Check sheet for the drawn part. Datum: minimum x, y, z corner. Units: mm. A direction names the side the tool comes from. Round coordinates to 2 decimals unless told otherwise and drop trailing zeros. Write each loop counter-clockwise with the first axis right and the second up, starting at its lowest first coordinate (ties: lowest second). Pieces come first, ordered by that corner, then holes. Notation, with made-up numbers: (0, 52.5) -> (18, 52.5) arc R35 ccw to (18, 86.5) -> close; hole circle Ø11 at (47, 50). An arc over 180 degrees is marked (long way). One line per item, written item: value.
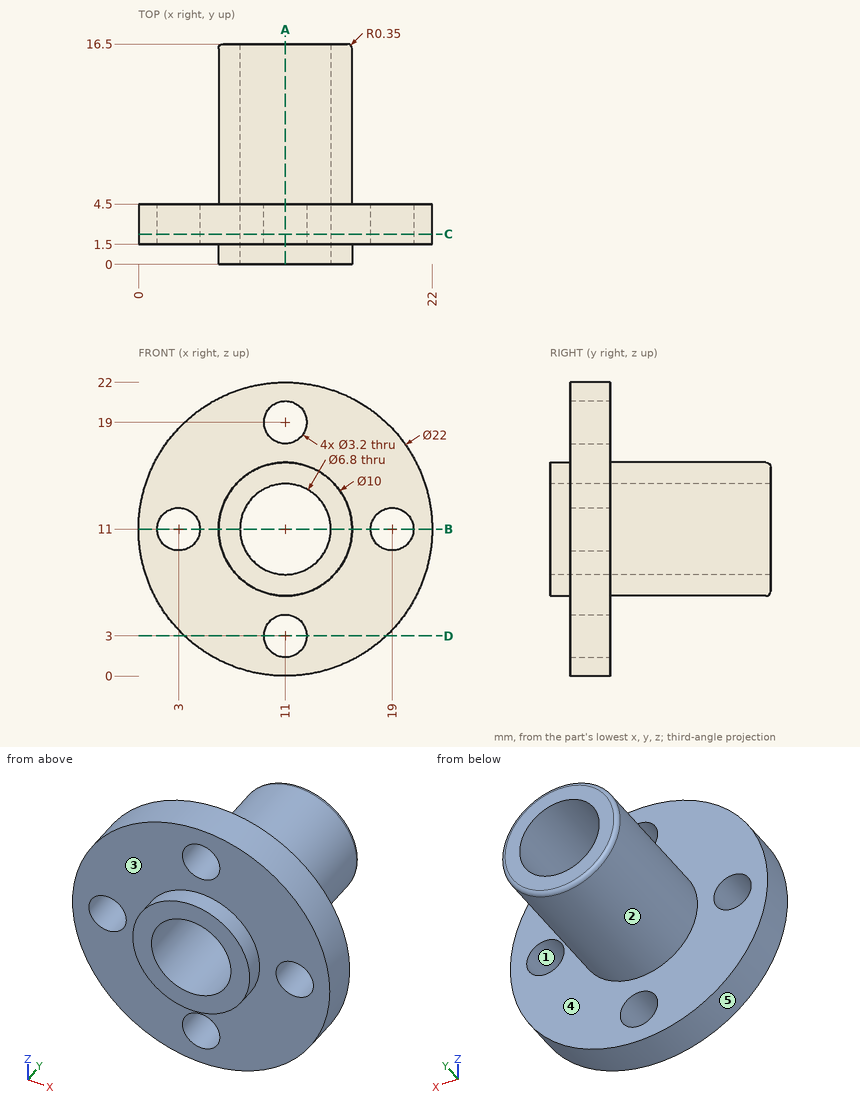
Item 1: Thickness scan on line 1 (Z direction, x = 11, y = 2.45); line 2 (X direction, y = 2.3, z = 3). Record the ranges inside material, lowest first.
Answer:
line 1: z = 0 to 1.4, 4.6 to 7.6, 14.4 to 17.4, 20.6 to 22
line 2: x = 3.45 to 9.4, 12.6 to 18.55
Item 2: Depth check by flat-ended pin: P1, Ø4, axis at x = 2.5, z = 7.5, coming from the -Y side; P2, Ø3, axis at x = 11, z = 3, coming from the +Y side; P3, Ø1, axis at y = 6, z = 15.5, coming from the +X side; P4, Ø3, axis at x = 9, z = 4, coming from the +Y side. Enter the tip coordinate at first touch or a pass-through.
Answer:
P1: stops at y = 1.5
P2: passes through
P3: stops at x = 14
P4: stops at y = 4.5
Item 3: Tool access check on the marked faces 4 and 5. Record the directions out of +Z, -Z, +X, -X, +Y, -Y that give a thin tool (end or side, any length) a straight path to the whole face; none if there is none.
Answer:
face 4: +Y
face 5: +Y, -Y
Item 4: Sectioned sample at A-A on x = 11. Enter the section's corners in (y, z).
Answer:
outline: (0, 6) -> (1.5, 6) -> (1.5, 4.6) -> (4.5, 4.6) -> (4.5, 6) -> (16.15, 6) arc R0.35 ccw to (16.5, 6.35) -> (16.5, 7.6) -> (0, 7.6) -> close; (0, 14.4) -> (16.5, 14.4) -> (16.5, 15.65) arc R0.35 ccw to (16.15, 16) -> (4.5, 16) -> (4.5, 17.4) -> (1.5, 17.4) -> (1.5, 16) -> (0, 16) -> close; (1.5, 0) -> (4.5, 0) -> (4.5, 1.4) -> (1.5, 1.4) -> close; (1.5, 20.6) -> (4.5, 20.6) -> (4.5, 22) -> (1.5, 22) -> close
Item 5: Sectioned sample at C-C on y = 2.25. Enter the section's corners in (x, z), and give its area (3 significant figures).
Answer:
outline: circle Ø22 at (11, 11); hole circle Ø3.2 at (3, 11); hole circle Ø6.8 at (11, 11); hole circle Ø3.2 at (11, 3); hole circle Ø3.2 at (11, 19); hole circle Ø3.2 at (19, 11)
area: 312 mm^2
Item 6: Mould release check, pull along Z, two halves, no side actions. Record for the marked faces 1, 2 and 3: pulls with the +Z half, pulls with the -Z half, needs draft (parallel to the pull), parting line crosses it, or undercut.
Answer:
face 1: undercut
face 2: parting line crosses it
face 3: needs draft
Item 7: Sectioned sample at B-B on z = 11. Enter the section's corners in (x, y), and give its area (3 significant figures).
Answer:
outline: (0, 1.5) -> (1.4, 1.5) -> (1.4, 4.5) -> (0, 4.5) -> close; (4.6, 1.5) -> (6, 1.5) -> (6, 0) -> (7.6, 0) -> (7.6, 16.5) -> (6.35, 16.5) arc R0.35 ccw to (6, 16.15) -> (6, 4.5) -> (4.6, 4.5) -> close; (14.4, 0) -> (16, 0) -> (16, 1.5) -> (17.4, 1.5) -> (17.4, 4.5) -> (16, 4.5) -> (16, 16.15) arc R0.35 ccw to (15.65, 16.5) -> (14.4, 16.5) -> close; (20.6, 1.5) -> (22, 1.5) -> (22, 4.5) -> (20.6, 4.5) -> close
area: 69.5 mm^2
Item 8: Sectioned sample at D-D on z = 3. Enter the section's corners in (x, y).
Answer:
outline: (3.45, 1.5) -> (9.4, 1.5) -> (9.4, 4.5) -> (3.45, 4.5) -> close; (12.6, 1.5) -> (18.55, 1.5) -> (18.55, 4.5) -> (12.6, 4.5) -> close
